```python
from build123d import *

# Parameters (mm, degrees)
SKETCH1_W           = 60
SKETCH1_H           = 40
BOSS_EXTRUDE1_DEPTH = 15
CUT_EXTRUDE1_REACH  = 17
SKETCH2_R           = 7.5
CUT_EXTRUDE2_REACH  = 17
SKETCH3_W           = 20
SKETCH3_H           = 20


with BuildPart() as part:
    # Sketch1 → Boss-Extrude1 (new body)
    with BuildSketch(Plane(origin=(0, 0, 0), x_dir=(1, 0, 0), z_dir=(0, 1, 0))):
        Rectangle(SKETCH1_W, SKETCH1_H)
    extrude(amount=BOSS_EXTRUDE1_DEPTH)

    # Sketch2 → Cut-Extrude1 (cut, up to next)
    with BuildSketch(Plane(origin=(0, 15, 0), x_dir=(1, 0, 0), z_dir=(0, 1, 0)), mode=Mode.PRIVATE) as cut_extrude1_sk1:
        with Locations((-15, 0)):
            Circle(SKETCH2_R)
    cut_extrude1_tool1 = extrude(cut_extrude1_sk1.sketch, amount=-CUT_EXTRUDE1_REACH, mode=Mode.PRIVATE) & part.part
    add(cut_extrude1_tool1.solids().sort_by_distance((-15, 15, 0))[0], mode=Mode.SUBTRACT)

    # Sketch3 → Cut-Extrude2 (cut, up to next)
    with BuildSketch(Plane(origin=(0, 15, 0), x_dir=(1, 0, 0), z_dir=(0, 1, 0)), mode=Mode.PRIVATE) as cut_extrude2_sk1:
        with Locations((20, 0)):
            Rectangle(SKETCH3_W, SKETCH3_H)
    cut_extrude2_tool1 = extrude(cut_extrude2_sk1.sketch, amount=-CUT_EXTRUDE2_REACH, mode=Mode.PRIVATE) & part.part
    add(cut_extrude2_tool1.solids().sort_by_distance((20, 15, 0))[0], mode=Mode.SUBTRACT)


solid = part.part
```
Can you work these out from the model? Positions are in its coordinate system, mm. A direction names the side the tool comes from. Give positions to 0.01 mm unless a question says otherwise; leave off trailing zeros. Loops run counter-clockwise (first coordinate to the right, second up) from the corner with the lowest first, then second, coordinate; pieces in that order, holes last. Notation, with made-up numbers: M -12.75,15.25 L 22.25,15.25 A25 ccw 22.25,37.25 Z; hole C -22.5,40 d10. An arc over 180 degrees is marked long. Answer in a Markdown table with one row per item.
1. If I drill on line 1 along Z through (x, y) = (-15, 7.25); line 2 along X through (y, z) = (11.25, 0); line 3 along X through (y, z) = (8.5, -5), over which ranges is the centre line in solid material (lowest first)?
Taken from the geometry:
| item | result |
|---|---|
| line 1 | z = -20 to -7.5, 7.5 to 20 |
| line 2 | x = -30 to -22.5, -7.5 to 10 |
| line 3 | x = -30 to -20.59, -9.41 to 10 |
2. Suppose I cut it at A-A on x = -15. Write out the boundary of the cut face in (y, z), plus the area to 3 significant figures.
Taken from the geometry:
| item | result |
|---|---|
| outline | M 0,-20 L 15,-20 L 15,-7.5 L 0,-7.5 Z; M 0,7.5 L 15,7.5 L 15,20 L 0,20 Z |
| area | 375 mm² |
3. Suppose I cut it at B-B on z = 0. Write out the boundary of the cut face in (x, y).
Taken from the geometry:
| item | result |
|---|---|
| outline | M -30,0 L -22.5,0 L -22.5,15 L -30,15 Z; M -7.5,0 L 10,0 L 10,15 L -7.5,15 Z |
4. Which directions (+Z, -Z, +X, -X, +Y, -Y) give clear straight access to the entire face, cutting with the end or side of a thin tool? Please do faces 1 (the flat face through (30, 7, -15)), 2 (the flat face through (20, 8, -10)).
Taken from the geometry:
| item | result |
|---|---|
| face 1 | +Z, -Z, +X, +Y, -Y |
| face 2 | +X, +Y, -Y |
5. Suppose I cut it at C-C on y = 4.5. Write out the boundary of the cut face in (x, z).
Taken from the geometry:
| item | result |
|---|---|
| outline | M -30,-20 L 30,-20 L 30,-10 L 10,-10 L 10,10 L 30,10 L 30,20 L -30,20 Z; hole C -15,0 d15 |
6. Thinking about a two-plate mould opening in Z: for faces 3 (the flat face through (30, 7, 15)), 4 (the flat face through (10, 8, 0)), 5 (the flat face through (0, 7, 20)), which applies, released by +Z, released by -Z, zero draft, split by the parting line, or undercut?
Taken from the geometry:
| item | result |
|---|---|
| face 3 | zero draft |
| face 4 | undercut |
| face 5 | released by +Z |
7. For pin 1 Ø7.5 at (y, z) = (8, 1) entering from +X, with a flat end and sliding along its axis, tell me the tip position at first contact or that it passes through.
Taken from the geometry:
| item | result |
|---|---|
| pin 1 | stops at x = 10 |
8. Suppose I cut it at D-D on z = 9. Write out the boundary of the cut face in (x, y), plus the area to 3 significant figures.
Taken from the geometry:
| item | result |
|---|---|
| outline | M -30,0 L 10,0 L 10,15 L -30,15 Z |
| area | 600 mm² |
